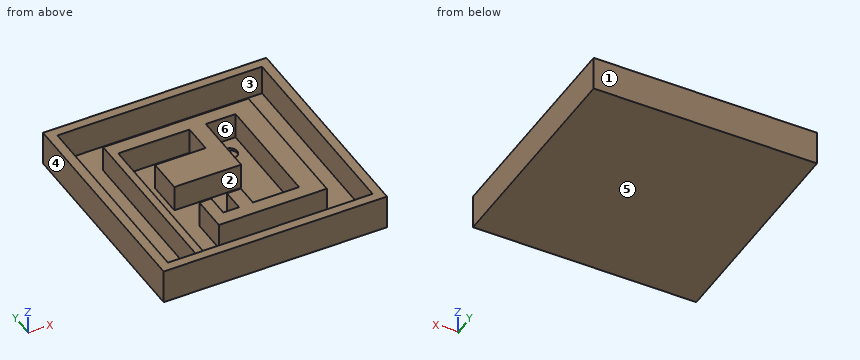
```python
from build123d import *

# Parameters (mm, degrees)
F0_W      = 38.1
F0_H      = 38.1
F1_DEPTH  = 0.79375
F2_W      = 38.1
F2_H      = 38.1
F2_W_2    = 34.925
F2_H_2    = 34.925
F3_DEPTH  = 5.08
F6_DEPTH  = 1.5875
F7_W      = 8.6149428158
F7_H      = 6.0720914678
F7_W_2    = 2.3730299118
F7_H_2    = 3.8083838299
F7_W_3    = 2.0170976641
F8_DEPTH  = 4.445
F9_R      = 1.2241603382
F9_R_2    = 1.27
F10_DEPTH = 0.396875
F11_DEPTH = 0.2286
F12_DEPTH = 1.8161


with BuildPart() as f1:
    # F0 (on Top) → F1 (new body)
    with BuildSketch(Plane.XY):
        with Locations((2.3213718086, -3.6332369254)):
            Rectangle(F0_W, F0_H)
    extrude(amount=F1_DEPTH)

    # F2 (on face) → F3 (join)
    with BuildSketch(Plane.XY.offset(0.79375)):
        with Locations((2.3213718086, -3.6332369254)):
            Rectangle(F2_W, F2_H)
        with Locations((2.3213718086, -3.6332369254)):
            Rectangle(F2_W_2, F2_H_2, mode=Mode.SUBTRACT)
    extrude(amount=F3_DEPTH)

    # F4 (on face) → F6 (join)
    with BuildSketch(Plane.XY.offset(0.79375)):
        Polygon((-10.0611281914, 8.7492630746), (-10.0611281914, -21.0957369254), (-8.7911281914, -21.0957369254), (-8.7911281914, 6.362864282), (3.3684632859, 6.362864282), (3.3684632859, -4.7892271858), (6.1505037943, -4.7892271858), (6.1505037943, 6.362864282), (12.7729084343, 6.362864282), (14.7038718086, 6.362864282), (14.7038718086, 8.7492630746), (-8.7911281914, 8.7492630746), align=None)
    extrude(amount=F6_DEPTH)

    # F7 (on face) + F6_face (on face) → F8 (join)
    with BuildSketch(Plane.XY.offset(0.79375)):
        with Locations((-0.939008122, -1.7531814519)):
            Rectangle(F7_W, F7_H)
        Polygon((14.7038718086, -16.0157369254), (14.7038718086, 6.362864282), (11.2305037943, 6.362864282), (11.2305037943, -13.6776110157), (11.2305037943, -16.0157369254), align=None)
        Polygon((11.2305037943, -16.0157369254), (11.2305037943, -13.6776110157), (3.3684632859, -13.6776110157), (0.995433374, -13.6776110157), (-1.6940305273, -13.6776110157), (-3.7111281914, -13.6776110157), (-3.7111281914, -16.0157369254), align=None)
        with Locations((2.18194833, -11.7734191008)):
            Rectangle(F7_W_2, F7_H_2)
        with Locations((-2.7025793593, -11.7734191008)):
            Rectangle(F7_W_3, F7_H_2)
    with BuildSketch(Plane(origin=(-0.3508488173, 1.7127034678, 2.38125), x_dir=(1, 0, 0), z_dir=(0, 0, 1))):
        Polygon((15.054720626, 7.0365596068), (-9.710279374, 7.0365596068), (-9.710279374, -22.8084403932), (-8.440279374, -22.8084403932), (-8.440279374, 4.6501608142), (3.7193121032, 4.6501608142), (3.7193121032, -6.5019306536), (6.5013526117, -6.5019306536), (6.5013526117, 4.6501608142), (15.054720626, 4.6501608142), align=None)
    extrude(amount=F8_DEPTH)

    # F9 (on face) → F10 (cut)
    with BuildSketch(Plane.XY.offset(0.79375)):
        with Locations((-12.3845431954, -17.3266101629)):
            Circle(F9_R)
        with Locations((8.5934712139, 3.3424642536)):
            Circle(F9_R_2)
    extrude(amount=-F10_DEPTH, mode=Mode.SUBTRACT)

    # F11 (add): a face of the model
    f11_faces = [f1.faces().sort_by_distance(p)[0] for p in [
        (2.3213718086, 8.3614449148, 6.82625),
    ]]
    extrude(f11_faces, amount=F11_DEPTH)

    # F12 (cut, through all): a face of the model
    f12_faces = [f1.faces().sort_by_distance(p)[0] for p in [
        (2.3213718086, 8.3614449148, 7.05485),
    ]]
    extrude(f12_faces, amount=-F12_DEPTH, mode=Mode.SUBTRACT)


solid = f1.part
```
The listing builds one solid part. Answer for the finished solid, in the listing's coordinates (mm). Face numbers are marked on the shaded views. A direction names the side the tool comes from. Give positions to 0.01 mm unless a question says otherwise; leave off trailing zeros. Order: outer loops, then holes, each group sorted by start corner. A loop starts at its lowest first (then second) coordinate and runs counter-clockwise, first axis right, second up. Notation, with made-up numbers: (19.25, 5) - (69.25, 5) arc R25 ccw to (69.25, 24) - close; hole circle Ø1 at (61, 30.5). An arc over 180 degrees is marked (long way). Answer in a Markdown table with one row per item. Add a question column.
Q1. Find the intervals of material crossed by line 1 along Y through (x, z) = (-0.5, 1.75); line 2 along X through (y, z) = (4.5, 4.45); line 3 along Y through (x, z) = (-4, 2.2), in increasing order. Write a range as [from, to].
Q2. Given P1, Ø3, axis at x = 8.5, y = 4, coming from the +Z side; P2, Ø17.5, axis at x = 5, y = -12, coming from the +Z side, each flat-ended and moving along its own axis, determine where each tip first touches the part or whether it passes through.
Q3. The part is cut by section C-C (y = 0.5). Determine the outline of the cut face in (x, z), then the cut area to 3 significant figures.
Q4. Which of the six approach directions +Z, -Z, +X, -X, +Y, -Y give full straight-line access (tool end or side, diameter ignored) to the marked faces 5 and 6?
Q5. For a pull along X with two mould halves and no side action, classify the marked faces 1, 2, 3 and 4 as released by +X, released by -X, zero draft, split by the parting line, or undercut.
Q6. The part is cut by section D-D (x = -6.5). Determine the outline of the cut face in (y, z).
Q7. The part is cut by section B-B (x = 16.5). Determine the outline of the cut face in (y, z).
Determined:
| question | item | result |
|---|---|---|
| 1 | line 1 | y = [-22.68, -21.1], [-16.02, -13.68], [-4.79, 1.28], [6.36, 8.75], [13.83, 15.42] |
| 1 | line 2 | x = [-16.73, -15.14], [-10.06, -8.79], [3.37, 6.15], [11.23, 14.7], [19.78, 21.37] |
| 1 | line 3 | y = [-22.68, -21.1], [-4.79, 1.28], [6.36, 8.75], [13.83, 15.42] |
| 2 | P1 | stops at z = 0.79 |
| 2 | P2 | stops at z = 5.24 |
| 3 | outline | (-16.73, 0) - (21.37, 0) - (21.37, 5.87) - (19.78, 5.87) - (19.78, 0.79) - (14.7, 0.79) - (14.7, 5.24) - (11.23, 5.24) - (11.23, 0.79) - (6.15, 0.79) - (6.15, 5.24) - (-5.25, 5.24) - (-5.25, 0.79) - (-8.79, 0.79) - (-8.79, 5.24) - (-10.06, 5.24) - (-10.06, 0.79) - (-15.14, 0.79) - (-15.14, 5.87) - (-16.73, 5.87) - close |
| 3 | area | 118 mm² |
| 4 | face 5 | -Z, +X, -X, +Y, -Y |
| 4 | face 6 | +Z |
| 5 | face 1 | zero draft |
| 5 | face 2 | undercut |
| 5 | face 3 | undercut |
| 5 | face 4 | released by -X |
| 6 | outline | (-22.68, 0) - (15.42, 0) - (15.42, 5.87) - (13.83, 5.87) - (13.83, 0.79) - (8.75, 0.79) - (8.75, 5.24) - (6.36, 5.24) - (6.36, 0.79) - (-21.1, 0.79) - (-21.1, 5.87) - (-22.68, 5.87) - close |
| 7 | outline | (-22.68, 0) - (15.42, 0) - (15.42, 5.87) - (13.83, 5.87) - (13.83, 0.79) - (-21.1, 0.79) - (-21.1, 5.87) - (-22.68, 5.87) - close |
